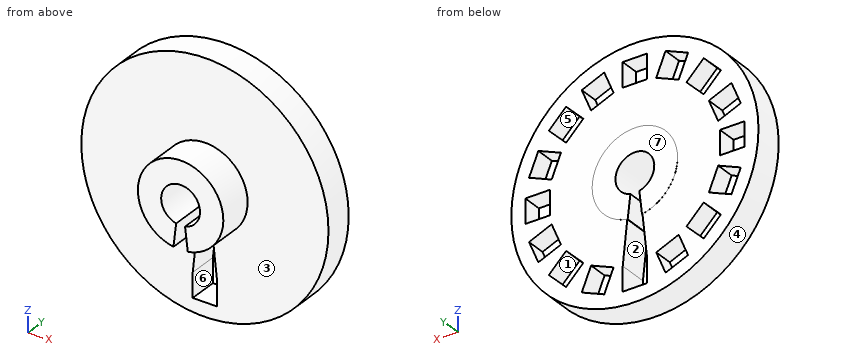
from build123d import *

# Parameters (mm, degrees)
SKETCH1_R                = 63.5
BOSS_EXTRUDE1_DEPTH      = 14.973360437
SKETCH2_W                = 12.5
SKETCH2_H                = 12.56
CUT_EXTRUDE1_DEPTH       = 10
CIRPATTERN1_COUNT        = 16
SKETCH5_W                = 12.5
SKETCH5_H                = 12.56
CUT_EXTRUDE3_DEPTH       = 37
CUT_EXTRUDE3_DEPTH_BACK  = 31
SKETCH6_R                = 17.625930659
CUT_EXTRUDE4_DEPTH       = 26
CUT_EXTRUDE4_DEPTH_BACK  = 37
CUT_EXTRUDE9_DEPTH       = 19
CUT_EXTRUDE9_DEPTH_BACK  = 11
SKETCH13_R               = 21.952850423
BOSS_EXTRUDE4_DEPTH      = 15
BOSS_EXTRUDE4_DEPTH_BACK = 18
SKETCH16_R               = 9.976383377
CUT_EXTRUDE11_DEPTH      = 33
CUT_EXTRUDE11_DEPTH_BACK = 29
CUT_EXTRUDE15_DEPTH      = 27
CUT_EXTRUDE15_DEPTH_BACK = 29


with BuildPart() as part:
    # Sketch1 → Boss-Extrude1 (new body)
    with BuildSketch(Plane(origin=(0, 0, 0), x_dir=(1, 0, 0), z_dir=(0, 1, 0))):
        Circle(SKETCH1_R)
    extrude(amount=BOSS_EXTRUDE1_DEPTH)

    # Sketch2 → Cut-Extrude1 (cut)
    with BuildSketch(Plane(origin=(0, 14.973360437, 0), x_dir=(1, 0, 0), z_dir=(0, 1, 0))):
        with Locations((0, -50)):
            Rectangle(SKETCH2_W, SKETCH2_H)
    cut_extrude1 = extrude(amount=-CUT_EXTRUDE1_DEPTH, mode=Mode.SUBTRACT)

    # CirPattern1: Cut-Extrude1 ×16 about axis
    cirpattern1_axis = Axis((0, 0, 0), (0, 1, 0))
    for i in range(1, CIRPATTERN1_COUNT):
        add(cut_extrude1.rotate(cirpattern1_axis, i * 360 / CIRPATTERN1_COUNT), mode=Mode.SUBTRACT)

    # Sketch5 → Cut-Extrude3 (cut, two sides)
    with BuildSketch(Plane(origin=(0, 0, 0), x_dir=(1, 0, 0), z_dir=(0, 1, 0))) as cut_extrude3_sk:
        with Locations((0, 50)):
            Rectangle(SKETCH5_W, SKETCH5_H)
    extrude(amount=CUT_EXTRUDE3_DEPTH, mode=Mode.SUBTRACT)
    extrude(cut_extrude3_sk.sketch, amount=-CUT_EXTRUDE3_DEPTH_BACK, mode=Mode.SUBTRACT)

    # Sketch6 → Cut-Extrude4 (cut, two sides)
    with BuildSketch(Plane(origin=(0, 14.973360437, 0), x_dir=(1, 0, 0), z_dir=(0, 1, 0))) as cut_extrude4_sk:
        Circle(SKETCH6_R)
    extrude(amount=CUT_EXTRUDE4_DEPTH, mode=Mode.SUBTRACT)
    extrude(cut_extrude4_sk.sketch, amount=-CUT_EXTRUDE4_DEPTH_BACK, mode=Mode.SUBTRACT)

    # Sketch9 → Cut-Extrude9 (cut, two sides)
    with BuildSketch(Plane(origin=(0, 0, 0), x_dir=(1, 0, 0), z_dir=(0, 1, 0))) as cut_extrude9_sk:
        Polygon((-6.25, 43.72), (0, -15.098638444), (6.25, 43.72), align=None)
    extrude(amount=CUT_EXTRUDE9_DEPTH, mode=Mode.SUBTRACT)
    extrude(cut_extrude9_sk.sketch, amount=-CUT_EXTRUDE9_DEPTH_BACK, mode=Mode.SUBTRACT)

    # Sketch13 → Boss-Extrude4 (add, two sides)
    with BuildSketch(Plane(origin=(0, 0, 0), x_dir=(1, 0, 0), z_dir=(0, 1, 0))) as boss_extrude4_sk:
        Circle(SKETCH13_R)
    extrude(amount=BOSS_EXTRUDE4_DEPTH)
    extrude(boss_extrude4_sk.sketch, amount=-BOSS_EXTRUDE4_DEPTH_BACK)

    # Sketch16 → Cut-Extrude11 (cut, two sides)
    with BuildSketch(Plane(origin=(0, 0, 0), x_dir=(1, 0, 0), z_dir=(0, 1, 0))) as cut_extrude11_sk:
        Circle(SKETCH16_R)
    extrude(amount=CUT_EXTRUDE11_DEPTH, mode=Mode.SUBTRACT)
    extrude(cut_extrude11_sk.sketch, amount=-CUT_EXTRUDE11_DEPTH_BACK, mode=Mode.SUBTRACT)

    # Sketch17 → Cut-Extrude15 (cut, two sides)
    with BuildSketch(Plane(origin=(0, 0, 0), x_dir=(1, 0, 0), z_dir=(0, 1, 0))) as cut_extrude15_sk:
        Polygon((-6.25, 43.72), (0, -9.976383377), (6.25, 43.72), align=None)
    extrude(amount=CUT_EXTRUDE15_DEPTH, mode=Mode.SUBTRACT)
    extrude(cut_extrude15_sk.sketch, amount=-CUT_EXTRUDE15_DEPTH_BACK, mode=Mode.SUBTRACT)


solid = part.part
Can you work these out from the model? Positions are in its coordinate system, mm. Face numbers are marked on the shaded views. A direction names the side the tool comes from. Round coordinates to 2 decimals unless told otherwise and drop trailing zeros. Use one line per item in the form item = value. Start each with the question number.
Q1. If I drill on probe 1 along Z at (x, y) = (0, 6); probe 2 along X at (y, z) = (12.5, -4.5); probe 3 along Z at (x, y) = (0, 1), over which ranges is the centre line in solid material (lowest first)? Write a range as [from, to].
Q2. I'm going to push flat-ended pins straight in: P1, Ø6.5, axis at y = 8, z = -50, coming from the +X side; P2, Ø2, axis at x = 16.5, y = -10, coming from the -Z side; P3, Ø4, axis at x = 41, z = 26.5, coming from the +Y side. Where does each tip first touch, or does it pass through?
Q3. Which directions (+Z, -Z, +X, -X, +Y, -Y) give clear straight access to the entire face, cutting with the end or side of a thin tool? Please do the marked faces 1, 2 and 3.
Q4. Imagine slicing it at C-C (y = 12). Count the separate pieces of the cut face and the enclosed holes in it, then the cut area to 3 significant figures.
Q5. We'd pull the mould along Z, two halves only. Please class the marked faces 4, 5, 6 and 7: +Z half, -Z half, draft (parallel to the pull), parting line (faces both ways), or undercut.
Worked out:
q1.probe_1 = [-63.5, -56.28], [9.98, 43.72], [56.28, 63.5]
q1.probe_2 = [-63.34, -56.28], [-43.72, -8.9], [8.9, 43.72], [56.28, 63.34]
q1.probe_3 = [-63.5, -56.28], [9.98, 63.5]
q2.P1 = 42.97
q2.P2 = -15.55
q2.P3 = 14.97
q3.face_1 = +Y
q3.face_2 = +Y, -Y
q3.face_3 = -Y
q4.separate_pieces = 1
q4.enclosed_holes = 16
q4.area = 9,550 mm^2
q5.face_4 = parting line
q5.face_5 = undercut
q5.face_6 = undercut
q5.face_7 = draft
